Could you check a few things on this model? Use its own coordinates, in mm. A direction names the side the tool comes from. Give positions to 0.01 mm unless a question says otherwise; leave off trailing zeros. Loops run counter-clockwise (first coordinate to the right, second up) from the corner with the lowest first, then second, coordinate; pieces in that order, holes last. Notation, with made-up numbers: (-38, -19.75) - (12, -19.75) arc R8 cw to (12, -8.75) - close; hole circle Ø1 at (46, 67). An arc over 180 degrees is marked (long way). Write each question's results on one line, items separated by ' | '. Start each with the question number.
1) On a 3-axis mill with a long thin cutter (end or side, diameter ignored), from which of +Z, -Z, +X, -X, +Y, -Y can I reach the whole of each face in a straight line? I mean faces 1 (the face through (-1, 0, 1.5)), 2 (the face through (45.66, 35.6, 1.48)). Say none if no direction works.
2) If I drill on probe 1 along Y at (x, z) = (44, 2.35); probe 2 along X at (y, z) = (-35, 2.5); probe 3 along X at (y, z) = (33.5, 2.1), over which ranges is the centre line in solid material (lowest first)? Write a range as [from, to].
3) I want a section at B-B, the plane x = -22.5. Write out the boundary of the cut face in (y, z).
4) I want a section at A-A, the plane y = 16. Write out the boundary of the cut face in (x, z), and give its area (3 significant figures).
5) If we mould it in two halves opening along Y, with no side actions, what happens to faces 3 (the face through (45.6, -35.77, 1.48)), 4 (the face through (-4, 33, 3)), 5 (the face through (-1, 40, 2))? For each: +Y half, -Y half, draft (parallel to the pull), parting line (faces both ways), or undercut.
6) I'm going to push flat-ended pins straight in: pin 1 (5 mm diameter, centred on x = 20.5, y = 7, fed in from +Z); pin 2 (6.5 mm diameter, centred on x = -43.75, y = 35, fed in from -Z); pin 3 (3 mm diameter, centred on x = -43.75, y = -35, fed in from +Z) (1 decimal). Where does each tip first touch, or does it pass through?
7) I want a section at C-C, the plane z = 2.5. Write out the boundary of the cut face in (x, y).
from build123d import *

# Parameters (mm, degrees)
SKETCH_W     = 100
SKETCH_H     = 80
SKETCH_R     = 2
PAD_DEPTH    = 3
SKETCH002_W  = 80
SKETCH002_H  = 60
POCKET_DEPTH = 1.5
FILLET_R     = 1
FILLET001_R  = 1
FILLET002_R  = 1
FILLET003_R  = 1


with BuildPart() as part:
    # Sketch → Pad (new body)
    with BuildSketch(Plane.XY):
        Rectangle(SKETCH_W, SKETCH_H)
        with Locations((-43.75305, -35.00244)):
            Circle(SKETCH_R, mode=Mode.SUBTRACT)
        with Locations((43.75305, 35.00244)):
            Circle(SKETCH_R, mode=Mode.SUBTRACT)
        with Locations((-43.75305, 35.00244)):
            Circle(SKETCH_R, mode=Mode.SUBTRACT)
        with Locations((43.75305, -35.00244)):
            Circle(SKETCH_R, mode=Mode.SUBTRACT)
    extrude(amount=PAD_DEPTH)

    # Sketch002 (on Face10 of Pad) → Pocket (cut)
    with BuildSketch(Plane.XY.offset(3)):
        Rectangle(SKETCH002_W, SKETCH002_H)
    extrude(amount=-POCKET_DEPTH, mode=Mode.SUBTRACT)

    # Fillet
    fillet_edges = [part.edges().sort_by_distance(p)[0] for p in [
        (0, -40, 0),
    ]]
    fillet(fillet_edges, radius=FILLET_R)

    # Fillet001
    fillet001_edges = [part.edges().sort_by_distance(p)[0] for p in [
        (0, 40, 0),
    ]]
    fillet(fillet001_edges, radius=FILLET001_R)

    # Fillet002
    fillet002_edges = [part.edges().sort_by_distance(p)[0] for p in [
        (-50, 0, 0),
    ]]
    fillet(fillet002_edges, radius=FILLET002_R)

    # Fillet003
    fillet003_edges = [part.edges().sort_by_distance(p)[0] for p in [
        (50, 0, 0),
    ]]
    fillet(fillet003_edges, radius=FILLET003_R)


solid = part.part
Answers:
1) face 1: +Z | face 2: +Z, -Z
2) probe 1: y = [-40, -36.99], [-33.02, 33.02], [36.99, 40] | probe 2: x = [-50, -45.75], [-41.75, 41.75], [45.75, 50] | probe 3: x = [-50, -45.07], [-42.43, 42.43], [45.07, 50]
3) outline: (-40, 1) arc R1 ccw to (-39, 0) - (39, 0) arc R1 ccw to (40, 1) - (40, 3) - (30, 3) - (30, 1.5) - (-30, 1.5) - (-30, 3) - (-40, 3) - close
4) outline: (-50, 1) arc R1 ccw to (-49, 0) - (49, 0) arc R1 ccw to (50, 1) - (50, 3) - (40, 3) - (40, 1.5) - (-40, 1.5) - (-40, 3) - (-50, 3) - close | area: 180 mm2
5) face 3: undercut | face 4: draft | face 5: +Y half
6) pin 1: stops at z = 1.5 | pin 2: stops at z = 0 | pin 3: passes through
7) outline: (-50, -39) arc R1 ccw to (-49, -40) - (49, -40) arc R1 ccw to (50, -39) - (50, 39) arc R1 ccw to (49, 40) - (-49, 40) arc R1 ccw to (-50, 39) - close; hole circle Ø4 at (-43.75, -35); hole circle Ø4 at (-43.75, 35); hole (-40, -30) - (40, -30) - (40, 30) - (-40, 30) - close; hole circle Ø4 at (43.75, -35); hole circle Ø4 at (43.75, 35)
